Geometry: see drawing. Coordinates: mm, zero at the bounding-box minimum. A direction names the side the tool comes from. Round coordinates to 2 decimals unless told otherwise and drop trailing zeros. Write each loop counter-clockwise with the first axis right and the second up, starting at its lowest first coordinate (ties: lowest second). Pieces come first, ordered by that corner, then holes. Notation, with made-up numbers: M 10,6.5 L 14,6.5 A22 cw 14,16.5 Z; hole C -24,80.25 d3. An arc over 180 degrees is marked long. Use one line per item in the form item = value. Start each with the question number.
Item 1: Pin query (flat end, axial travel): pin 1 Ø3 at (x, z) = (5, 4) entering from +Y; pin 2 Ø4.5 at (x, y) = (8, 8) entering from -Z; pin 3 Ø1.5 at (y, z) = (2.5, 4) entering from +X; pin 4 Ø3 at (x, z) = (13, 3) entering from -Y. Return the tip coordinate at first contact, or that it passes through.
Item 2: Ray query, probe 1 along Y at (x, z) = (8, 4.9) (1 decimal); probe 2 along Y at (x, z) = (8, 0.25); probe 3 along Z at (x, y) = (12.5, 9.75). Return the intervals inside material, ascending.
Item 3: Section query D-D (y = 14.5). Return loops of the section in (x, z).
Item 4: Pull-direction query (Y, two-part tool) for the marked faces 1, 2 and 3; classes: pulls with the +Y half, pulls with the -Y half, needs draft (parallel to the pull), parting line crosses it, or undercut.
Item 5: Reachability of the marked faces 4 and 5 from +Z, -Z, +X, -X, +Y, -Y: full face, straight path, thin tool, end or side. Return the list, or none.
Item 6: Section query C-C (z = 3.6). Return loops of the section in (x, y), and give its area (3 significant figures).
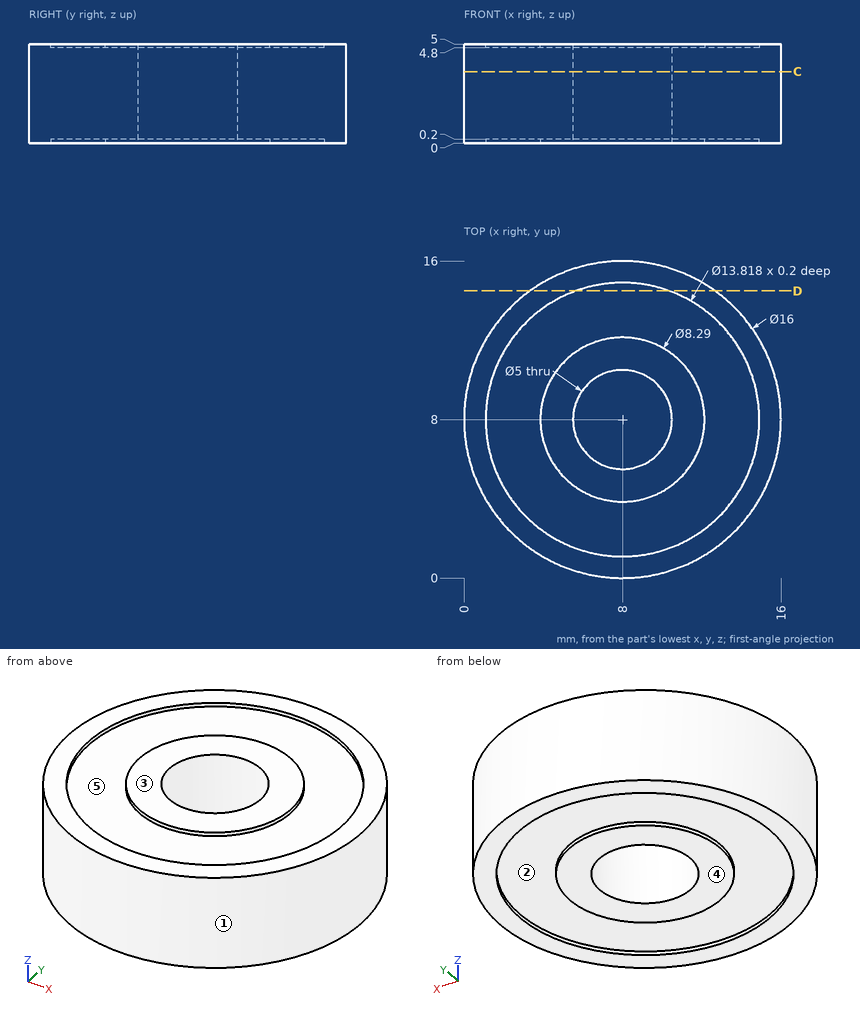
Working result:
q1.pin_1 = 15.86
q1.pin_2 = through
q1.pin_3 = 14.44
q1.pin_4 = 0.81
q2.probe_1 = 0 to 1.1, 3.9 to 5.5, 10.5 to 12.1, 14.9 to 16
q2.probe_2 = 0 to 5.5, 10.5 to 16
q2.probe_3 = 0.2 to 4.8
q3.outline = M 3.34,0 L 5.66,0 L 5.66,0.2 L 10.34,0.2 L 10.34,0 L 12.66,0 L 12.66,5 L 10.34,5 L 10.34,4.8 L 5.66,4.8 L 5.66,5 L 3.34,5 Z
q4.face_1 = parting line crosses it
q4.face_2 = undercut
q4.face_3 = needs draft
q5.face_4 = -Z, +X, -X, +Y, -Y
q5.face_5 = +Z
q6.outline = C 8,8 d16; hole C 8,8 d5
q6.area = 181 mm²
